For this review, take the finished solid that the model builds, in its own axes (mm). A direction names the side the tool comes from. Coordinates: 2 decimals unless noted, no trailing zeros. Order: outer loops, then holes, each group sorted by start corner. A loop starts at its lowest first (then second) coordinate and runs counter-clockwise, first axis right, second up. Notation, with made-up numbers: M -9,29.5 L 48,29.5 A23 ccw 48,62.5 Z; hole C 40.5,-3.75 d1. An arc over 180 degrees is marked long. Use CSV: the item, a comma, the result in double quotes.
Autodesk Fusion 360 part; units mm, degrees
sketch "Sketch1" plane through (0, 0, 0) normal (1, 0, 0) x (0, 0, -1)
  line L0 (0, 0) -> (0, 28)
  line L1 (0, 28) -> (5, 28)
  line L2 (6, 27) -> (6, 22)
  line L3 (6, 22) -> (22, 6)
  line L4 (22, 6) -> (27, 6)
  line L5 (28, 5) -> (28, 0)
  line L6 (28, 0) -> (0, 0)
  line L7 (4, 4) -> (28, 4)
  line L8 (4, 4) -> (4, 28)
  arc A0 (6, 27) -> (5, 28) centre (5, 27) ccw
  arc A1 (28, 5) -> (27, 6) centre (27, 5) ccw
  line L9 (0, 26.5) -> (-1.6, 24.9)
  line L10 (-1.6, 24.9) -> (-1.6, 23.5)
  line L11 (-1.6, 23.5) -> (0, 23.5)
  line L12 (0, 6.5) -> (-1.6, 4.9)
  line L13 (-1.6, 4.9) -> (-1.6, 3.5)
  line L14 (-1.6, 3.5) -> (0, 3.5)
  line L15 (3.5, 0) -> (3.5, -1.6)
  line L16 (3.5, -1.6) -> (4.9, -1.6)
  line L17 (4.9, -1.6) -> (6.5, 0)
  line L18 (23.5, 0) -> (23.5, -1.6)
  line L19 (23.5, -1.6) -> (24.9, -1.6)
  line L20 (24.9, -1.6) -> (26.5, 0)
  line L21 (-56.6063, 27.9695) -> (-36.6063, 27.9695)
  line L22 (-36.6063, 27.9695) -> (-36.6063, -0.0305)
  line L23 (-36.6063, -0.0305) -> (-56.6063, -0.0305)
  line L24 (-56.6063, -0.0305) -> (-56.6063, 27.9695)
  line L25 (-54.1063, 3.9695) -> (-39.1063, 3.9695)
  line L26 (-39.1063, 3.9695) -> (-39.1063, 27.9695)
  line L27 (-39.1063, 27.9695) -> (-54.1063, 27.9695)
  line L28 (-54.1063, 27.9695) -> (-54.1063, 3.9695)
  line L29 (-49.7743, 13.4695) -> (-49.7743, 16.9695)
  arc A2 (-43.2743, 16.9695) -> (-49.7743, 16.9695) centre (-46.5243, 16.9695) ccw
  line L30 (-43.2743, 16.9695) -> (-43.2743, 13.4695)
  arc A3 (-49.7743, 13.4695) -> (-43.2743, 13.4695) centre (-46.5243, 13.4695) ccw
  line L31 (-49.5243, -1.6305) -> (-43.5243, -1.6305)
  line L32 (-43.5243, -1.6305) -> (-43.5243, -0.0305)
  line L33 (-43.5243, -0.0305) -> (-49.5243, -0.0305)
  line L34 (-49.5243, -0.0305) -> (-49.5243, -1.6305)
  point P0 (6, 28)
  point P1 (28, 6)
  dimension "d1" = 28
  dimension "d2" = 28
  dimension "d3" = 6
  dimension "d4" = 6
  dimension "d5" = 45
  dimension "d6" = 22
  dimension "d7" = 4
  dimension "d8" = 4
  dimension "d9" = 1
  dimension "d11" = 45
  dimension "d12" = 1.6
  dimension "d14" = 3
  dimension "d16" = 3
  dimension "d17" = 20
  dimension "d18" = 20
  dimension "d19" = 3
  dimension "d20" = 3
  dimension "d21" = 45
  dimension "d22" = 3.5
  dimension "d23" = 1.6
  dimension "d26" = 20
  dimension "d27" = 2.5
  dimension "d28" = 15
  dimension "d29" = 6.5
  dimension "d30" = 3.5
  dimension "d31" = 13.5
  dimension "d32" = 4
  dimension "d33" = 28
  dimension "d34" = 6
  dimension "d35" = 0.25
  dimension "d36" = 1.6
  dimension "d41" = 3.5
extrude "Extrude1" add sketch "Sketch1" along normal mid plane 20 contours L0 L1 L5 L6 L7 L8 | L1 L2 L3 L4 L5 L7 L8 A0 A1
extrude "Extrude2" cut sketch "Sketch1" along normal mid plane 15 contours L1 L2 L3 L4 L5 L7 L8 A0 A1
extrude "Extrude3" add sketch "Sketch1" along normal mid plane 6 contours L0 L12 L13 L14 | L6 L15 L16 L17 | L0 L9 L10 L11 | L6 L18 L19 L20
sketch "Sketch2" plane through (0, 0, -4) normal (0, 0, -1) x (-1, 0, 0)
  line L0 (-7.5, 4) -> (7.5, 4)
  line L1 (7.5, 4) -> (7.5, 28)
  line L2 (7.5, 28) -> (-7.5, 28)
  line L3 (-7.5, 28) -> (-7.5, 4)
  line L4 (-3.25, 12.5) -> (-3.25, 18)
  arc A0 (3.25, 18) -> (-3.25, 18) centre (0, 18) ccw
  line L5 (3.25, 18) -> (3.25, 12.5)
  arc A1 (-3.25, 12.5) -> (3.25, 12.5) centre (0, 12.5) ccw
  line L6 (-10, 0) -> (10, 0)
  point P0 (0, 28)
  dimension "d42" = 6.5
  dimension "d43" = 5.5
  dimension "d44" = 12.5
extrude "Extrude4" cut sketch "Sketch2" against normal through all contours L4 A0 L5 A1
sketch "Sketch3" plane through (0, 4, 0) normal (0, 1, 0) x (-1, 0, 0)
  line L0 (-7.5, -28) -> (7.5, -28)
  line L1 (7.5, -28) -> (7.5, -4)
  line L2 (7.5, -4) -> (-7.5, -4)
  line L3 (-7.5, -4) -> (-7.5, -28)
  line L4 (3.25, -12.5) -> (3.25, -18)
  arc A0 (-3.25, -18) -> (3.25, -18) centre (0, -18) ccw
  line L5 (-3.25, -18) -> (-3.25, -12.5)
  arc A1 (3.25, -12.5) -> (-3.25, -12.5) centre (0, -12.5) ccw
  line L6 (10, 0) -> (-10, 0)
  point P0 (0, -28)
  dimension "d46" = 6.5
  dimension "d47" = 12.5
  dimension "d48" = 5.5
extrude "Extrude5" cut sketch "Sketch3" against normal through all contours L4 A0 L5 A1
equation "d16 = d14"
equation "d18 = d17"
equation "d19 = d14"
equation "d20 = d14"
equation "d21 = d11"
equation "d22 = d41"
equation "d23 = d12"
Item 1: Add section B-B on z = -13.25. State the section outline as (x, y) points.
Solutions:
outline,"M -10,0 L -3.25,0 L -3.25,4 L -7.5,4 L -7.5,14.75 L -10,14.75 Z; M 3.25,0 L 10,0 L 10,14.75 L 7.5,14.75 L 7.5,4 L 3.25,4 Z"
Item 2: Add section D-D on z = -4.5. State the section outline as (x, y) points.
Solutions:
outline,"M -10,0 L -3,0 L -3,-1.6 L 3,-1.6 L 3,0 L 10,0 L 10,28 L 7.5,28 L 7.5,4 L -7.5,4 L -7.5,28 L -10,28 Z"
Item 3: For faces 1 (the face through (-3, 25, 1)), 2 (the face through (-3.25, 2, -15)), 3 (the face through (-3.44, 15.83, -4)), 4 (the face through (9, 6, -24)), list the 3-axis set-ups (+Z, -Z, +X, -X, +Y, -Y) from which the entire face can be reached by the end or side of a thin tool; tool diameter is ignored.
Solutions:
face 1,"+Z, -X, +Y, -Y"
face 2,"+Y, -Y"
face 3,"-Z, +Y"
face 4,"-Z, +X, -X, +Y"
Item 4: To check wall thickness, follow line 1 along X through (y, z) = (8.25, -13.5); line 2 along X through (y, z) = (16.75, -2.75); line 3 along Z through (x, y) = (5.5, 25). State the ranges of each line that lie inside material, in increasing order. Write a range as [from, to].
Solutions:
line 1,"[-10, -7.5], [7.5, 10]"
line 2,"[-10, -3.25], [3.25, 10]"
line 3,"[-4, 0]"
Item 5: Add section A-A on x = 1.25. State how many separate pieces and enclosed holes the cut face has, and give its area (3 significant figures).
Solutions:
separate pieces,"3"
enclosed holes,"0"
area,"130 mm^2"
Item 6: Add section C-C on y = 7.25. State the section outline as (x, z) points, and give its area (3 significant figures).
Solutions:
outline,"M -10,-20.75 L -7.5,-20.75 L -7.5,-4 L 7.5,-4 L 7.5,-20.75 L 10,-20.75 L 10,0 L -10,0 Z"
area,"164 mm^2"
Item 7: Clearance check with flat-ended pins moving along their axes: pin 1 Ø6 at (x, y) = (3.5, 8.5) entering from -Z; pin 2 Ø1.3 at (y, z) = (25, 1) entering from +X; pin 3 Ø0.5 at (y, z) = (-1, -25) entering from -X; pin 4 Ø12 at (y, z) = (19, -19) entering from -X (3 decimals). State where each tip first meets the part, or that it passes through.
Solutions:
pin 1,"z = -4"
pin 2,"x = 3"
pin 3,"x = -3"
pin 4,"through"
Item 8: Draft analysis for pull direction Y (two halves, no side actions). For faces 5 (the face through (8.732, 5.715, -27.699)), 6 (the face through (3.25, 15, -2)), 7 (the face through (0, -0.8, -25.7)), 8 (the face through (-0.07, 21.25, -2.03)), state which applies: released by +Y, released by -Y, zero draft, split by the parting line, or undercut.
Solutions:
face 5,"released by +Y"
face 6,"undercut"
face 7,"released by -Y"
face 8,"undercut"
